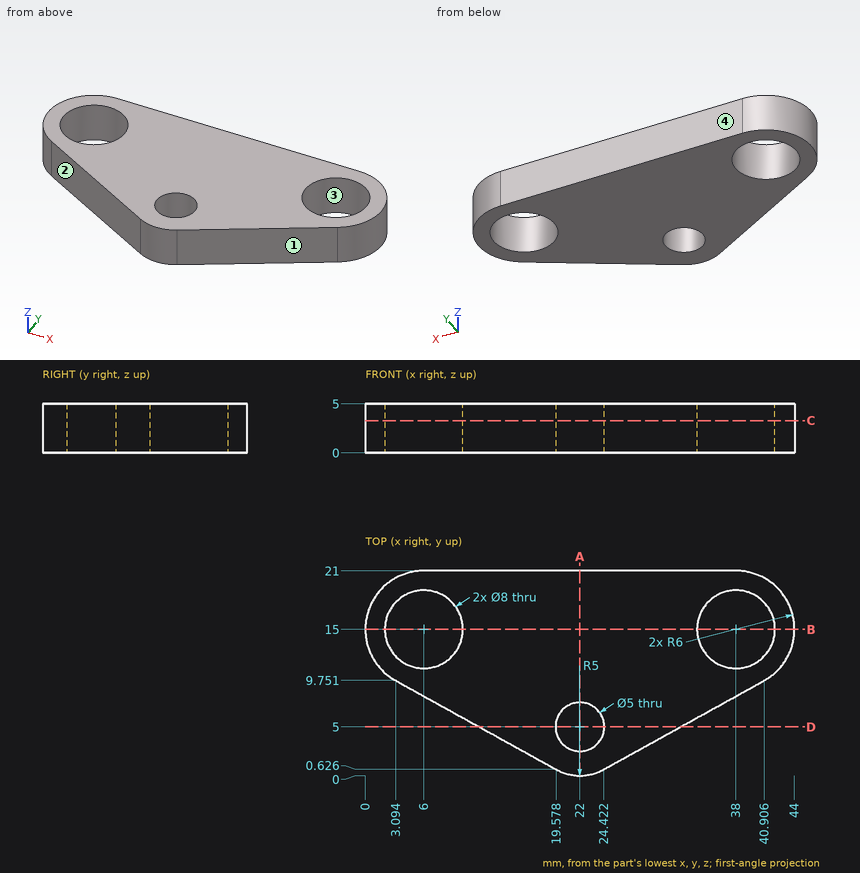
Answer from the drawing. Dimensions are ordinates in mm from the lowest x, y and z of the part. Coordinates: 2 decimals unless noted, no trailing zeros. Order: outer loops, then holes, each group sorted by start corner. A loop starts at its lowest first (then second) coordinate and runs counter-clockwise, first axis right, second up. Notation, with made-up numbers: M -40,55 L -17,55 A18 ccw -17,59 Z; hole C 4,-21 d10. An arc over 180 degrees is marked long. Put each result on its own line as item: value. Start each with the question number.
Item 1: Section A-A, the plane x = 22 is taken. Determine the outline of the cut face in (y, z).
Item 2: Given pin 1 Ø2 at (y, z) = (18.5, 3.5) entering from +X (1 decimal); pin 2 Ø2 at (x, z) = (8, 0.5) entering from -Y; pin 3 Ø10.5 at (x, y) = (38, 15) entering from -Z; pin 4 Ø3 at (x, z) = (27.5, 0.5) entering from -Y, each flat-ended and moving along its own axis, determine where each tip first touches the part or whether it passes through.
Item 3: Consider probe 1 along X at (y, z) = (13.5, 4.6); probe 2 along X at (y, z) = (18, 4.35) (1 decimal); probe 3 along Y at (x, z) = (41.5, 0.7) (1 decimal). Determine where each line is inside the solid, lowest interval first. Write a range as [from, to].
Item 4: Section D-D, the plane y = 5 is taken. Determine the outline of the cut face in (x, z).
Item 5: The mould has two halves that part along X. Classify the marked faces 1, 2, 3 and 4: +X half, -X half, draft (parallel to the pull), parting line (faces both ways), or undercut.
Item 6: Section C-C, the plane z = 3.3 is taken. Count the separate pieces of the cut face and the enclosed holes in it.
Item 7: Section B-B, the plane y = 15 is taken. Determine the outline of the cut face in (x, z).
Computed:
1. outline: M 0,0 L 2.5,0 L 2.5,5 L 0,5 Z; M 7.5,0 L 21,0 L 21,5 L 7.5,5 Z
2. pin 1: stops at x = 43.5
2. pin 2: stops at y = 6.48
2. pin 3: stops at z = 0
2. pin 4: stops at y = 1.5
3. probe 1: x = [0.19, 2.29], [9.71, 34.29], [41.71, 43.81]
3. probe 2: x = [0.8, 3.4], [8.6, 35.4], [40.6, 43.2]
3. probe 3: y = [10.1, 13.1], [16.9, 19.9]
4. outline: M 11.68,0 L 19.5,0 L 19.5,5 L 11.68,5 Z; M 24.5,0 L 32.32,0 L 32.32,5 L 24.5,5 Z
5. face 1: +X half
5. face 2: -X half
5. face 3: undercut
5. face 4: draft
6. separate pieces: 1
6. enclosed holes: 3
7. outline: M 0,0 L 2,0 L 2,5 L 0,5 Z; M 10,0 L 34,0 L 34,5 L 10,5 Z; M 42,0 L 44,0 L 44,5 L 42,5 Z
